Input: part model. Units: mm. Frame: model coordinates. A direction names the side the tool comes from. Give positions to 0.01 mm unless a question says otherwise; leave off trailing zeros. Loops run counter-clockwise (first coordinate to the right, second up) from the corner with the lowest first, then second, coordinate; pieces in that order, holes last. Notation, with made-up numbers: (63.25, 88.25) -> (101.25, 88.25) arc R17 ccw to (101.25, 110.25) -> close; hole circle Ø1 at (-8.5, 88). An arc over 180 degrees is marked (long way). Use CSV: the item, a comma, the result in double quotes.
```python
from build123d import *

# Parameters (mm, degrees)
BOSS_EXTRUDE1_REACH        = 163.827
BOSS_EXTRUDE1_START_RADIUS = 52.07
BOSS_EXTRUDE1_END_RADIUS   = 52.07
CIRPATTERN15_COUNT         = 20
SKETCH7_R                  = 3.81
CUT_EXTRUDE1_DEPTH         = 97.98975948


with BuildPart() as part:
    # Sketch1 → Revolve1 (revolve)
    with BuildSketch(Plane(origin=(0, 0, 0), x_dir=(1, 0, 0), z_dir=(0, 1, 0)), mode=Mode.PRIVATE) as revolve1_sk:
        Polygon((3.302, 0), (3.302, 50.8), (26.162, 50.8), (26.162, 52.07), (-6.35, 52.07), (-6.35, 50.8), (0, 50.8), (0, 0), align=None)
    revolve(revolve1_sk.sketch.rotate(Axis((0, 0, 0), (1, 0, 0)), 180), axis=Axis((0, 0, 0), (1, 0, 0)))

    # Boss-Extrude1: from a cylinder face, 163.827 long prism both ways, kept between that surface and its translate by the depth
    boss_extrude1_start = Plane(origin=(9.906, 0, 0), z_dir=(-1, 0, 0)) * Cylinder(BOSS_EXTRUDE1_START_RADIUS, 432.794, mode=Mode.PRIVATE)
    boss_extrude1_end = Plane(origin=(9.906, 0, 13.97), z_dir=(-1, 0, 0)) * Cylinder(BOSS_EXTRUDE1_END_RADIUS, 432.794, mode=Mode.PRIVATE)
    # Sketch2 → Boss-Extrude1 (add, from a surface)
    with BuildSketch(Plane.XY.offset(83.82), mode=Mode.PRIVATE) as boss_extrude1_sk1:
        Polygon((-2.974727154, -8.169926131), (23.421727154, 7.070073869), (22.786727154, 8.169926131), (-3.609727154, -7.070073869), align=None)
    boss_extrude1_tool1 = extrude(boss_extrude1_sk1.sketch, amount=BOSS_EXTRUDE1_REACH, both=True, mode=Mode.PRIVATE)
    boss_extrude1 = ((boss_extrude1_tool1 - boss_extrude1_start) & boss_extrude1_end).solids().sort_by_distance((9.906, 0, 58.491422))[0]
    add(boss_extrude1)

    # CirPattern15: Boss-Extrude1 ×20 about axis
    cirpattern15_axis = Axis((0, 0, 0), (1, 0, 0))
    for i in range(1, CIRPATTERN15_COUNT):
        add(boss_extrude1.rotate(cirpattern15_axis, i * 360 / CIRPATTERN15_COUNT))

    # Sketch7 → Cut-Extrude1 (cut, through all)
    with BuildSketch(Plane.ZY):
        Circle(SKETCH7_R)
    extrude(amount=-CUT_EXTRUDE1_DEPTH, mode=Mode.SUBTRACT)


solid = part.part
```
1) Mould query, pull axis Y, two halves, no side actions, for faces 6 (the flat face through (-3.297, -40.597, 42.926)), 7 (the flat face through (-3.297, 42.926, 40.597)), 8 (the cylindrical face through (9.84, 0.04, -66.04)), 9 (the flat face through (23.1, 40.6, 42.9)). Classes: pulls with the +Y half, pulls with the -Y half, needs draft (parallel to the pull), parting line crosses it, or undercut.
From the geometry:
face 6,"pulls with the -Y half"
face 7,"undercut"
face 8,"parting line crosses it"
face 9,"pulls with the +Y half"
2) Reachability of faces 1 (the flat face through (10.04, -17.56, -56.16)), 2 (the flat face through (0, -1, 11)), 3 (the flat face through (-3.3, 51.87, -28.28)), 4 (the flat face through (23.109, -25.345, -53.37)), 5 (the flat face through (23.11, -51.87, -28.28)) from +Z, -Z, +X, -X, +Y, -Y: full face, straight path, thin tool, end or side. Return the list, or none.
From the geometry:
face 1,"-Z, +X"
face 2,"-X"
face 3,"-X, +Y"
face 4,"+X"
face 5,"+X, -Y"
3) Section query A-A (z = 0). Return loops of the section in (x, y), then the cut area to 3 significant figures.
From the geometry:
outline,"(-6.35, -52.07) -> (8.64, -52.07) -> (8.64, -66.04) -> (11.18, -66.04) -> (11.18, -52.07) -> (26.16, -52.07) -> (26.16, -50.8) -> (3.3, -50.8) -> (3.3, -3.81) -> (0, -3.81) -> (0, -50.8) -> (-6.35, -50.8) -> close; (-6.35, 50.8) -> (0, 50.8) -> (0, 3.81) -> (3.3, 3.81) -> (3.3, 50.8) -> (26.16, 50.8) -> (26.16, 52.07) -> (11.18, 52.07) -> (11.18, 66.04) -> (8.64, 66.04) -> (8.64, 52.07) -> (-6.35, 52.07) -> close"
area,"464 mm^2"
4) Ray query, line 1 (Y direction, x = 1.85, z = 0); line 2 (Z direction, x = 23, y = 56.5); line 3 (Y direction, x = 17.5, z = 60.5). Return the intervals inside material, ascending.
From the geometry:
line 1,"y = -52.07 to -3.81, 3.81 to 52.07"
line 2,"z = -26.56 to -25.54, -7.8 to -6.83, 10.16 to 11.18, 31.41 to 32.61"
line 3,"y = -15.82 to -14.28, 3.65 to 5.12, 23.5 to 25.04"
5) Section query C-C (z = 29.5). Return loops of the section in (x, y), then the cut area to 3 significant figures.
From the geometry:
outline,"(-6.35, -42.91) -> (6.29, -42.91) -> (-3.61, -52.63) -> (-2.97, -54.5) -> (8.83, -42.91) -> (26.16, -42.91) -> (26.16, -41.36) -> (3.3, -41.36) -> (3.3, 41.36) -> (26.16, 41.36) -> (26.16, 42.91) -> (13.52, 42.91) -> (23.42, 52.63) -> (22.79, 54.5) -> (10.98, 42.91) -> (-6.35, 42.91) -> (-6.35, 41.36) -> (0, 41.36) -> (0, -41.36) -> (-6.35, -41.36) -> close"
area,"428 mm^2"
6) Contact query for flat-ended pins moving along their axis: pin 1 (3 mm diameter, centred on x = 9, y = 3.5, fed in from +Z); pin 2 (6 mm diameter, centred on x = 21.5, z = -46.5, fed in from +Y); pin 3 (1.5 mm diameter, centred on y = 14, z = 37.5, fed in from +X); pin 4 (6 mm diameter, centred on y = 0, z = 0, fed in from -X). Output: stop coordinate, or through.
From the geometry:
pin 1,"stops at z = 52.03"
pin 2,"stops at y = 49.59"
pin 3,"stops at x = 3.3"
pin 4,"passes through"
